from build123d import *

# Parameters (mm, degrees)
SKETCH2_R           = 11
SKETCH2_R_2         = 7
BOSS_EXTRUDE1_DEPTH = 4


with BuildPart() as part:
    # Sketch2 → Boss-Extrude1 (new body)
    with BuildSketch(Plane.XY):
        with BuildLine():
            Line((30.078103468, 30.102899094), (30.078103468, 104.858637586))
            Line((30.078103468, 104.858637586), (43.656234688, 145.478166756))
            Line((43.656234688, 145.478166756), (60.038536544, 194.486485935))
            Line((60.038536544, 194.486485935), (60.038536544, 254.427096014))
            ThreePointArc((60.038536544, 254.427096014), (45.05832001, 260.632104877), (30.078103469, 254.427096029))
            Line((30.078103469, 254.427096029), (22.62926434, 194.486485916))
            Line((22.62926434, 194.486485916), (-14.683335653, 89.230795609))
            Line((-14.683335653, 89.230795609), (-17.49123357, 0.553848547))
            ThreePointArc((-17.49123357, 0.553848547), (-3.415184823, -17.163522734), (16.370945819, -6.184022397))
            Line((16.370945819, -6.184022397), (30.078103468, 30.102899094))
        make_face()
        Circle(SKETCH2_R, mode=Mode.SUBTRACT)
        with Locations((45.058319997, 232.788133995)):
            Circle(SKETCH2_R_2, mode=Mode.SUBTRACT)
        with Locations((42.85515341, 200.574247039)):
            Circle(SKETCH2_R_2, mode=Mode.SUBTRACT)
        with Locations((32.877400798, 166.36480954)):
            Circle(SKETCH2_R_2, mode=Mode.SUBTRACT)
        with Locations((22.629264347, 133.284451418)):
            Circle(SKETCH2_R_2, mode=Mode.SUBTRACT)
        with Locations((10.792452444, 95.075946031)):
            Circle(SKETCH2_R_2, mode=Mode.SUBTRACT)
        with Locations((5.075535148, 44.712849864)):
            Circle(SKETCH2_R, mode=Mode.SUBTRACT)
    extrude(amount=BOSS_EXTRUDE1_DEPTH)


solid = part.part
Here's how the part is built. I have some questions about the finished solid (model axes, mm). Coordinates: 2 decimals unless noted, no trailing zeros. Order: outer loops, then holes, each group sorted by start corner. A loop starts at its lowest first (then second) coordinate and runs counter-clockwise, first axis right, second up.
Item 1: I need wall thicknesses on line 1 (X direction, y = 43, z = 0.2); line 2 (X direction, y = 130, z = 1.05); line 3 (X direction, y = 179.5, z = 0.2). Which ranges of each line are inside material? Lowest first, please.
Result sheet:
line 1: x = -16.15 to -5.79, 15.94 to 30.08
line 2: x = -0.23 to 16.45, 28.81 to 38.48
line 3: x = 17.32 to 55.03
Item 2: If we section it at D-D on x = -1: List the corners of the cut face in (y, z) for me, plus the area to 3 significant figures.
Result sheet:
outline: (-17.47, 0) - (-10.95, 0) - (-10.95, 4) - (-17.47, 4) - close; (10.95, 0) - (35.54, 0) - (35.54, 4) - (10.95, 4) - close; (53.88, 0) - (127.83, 0) - (127.83, 4) - (53.88, 4) - close
area: 420 mm2
Item 3: If we section it at A-A on x = 47: List the corners of the cut face in (y, z) for me, plus the area to 3 significant figures.
Result sheet:
outline: (155.48, 0) - (194.93, 0) - (194.93, 4) - (155.48, 4) - close; (206.22, 0) - (226.06, 0) - (226.06, 4) - (206.22, 4) - close; (239.51, 0) - (260.54, 0) - (260.54, 4) - (239.51, 4) - close
area: 321 mm2
Item 4: If we section it at C-C on y = 162: List the corners of the cut face in (x, z) for me.
Result sheet:
outline: (11.11, 0) - (27.4, 0) - (27.4, 4) - (11.11, 4) - close; (38.35, 0) - (49.18, 0) - (49.18, 4) - (38.35, 4) - close
Item 5: For P1, Ø1.2, axis at y = 53, z = 2, coming from the +X side, with a flat end and sliding along its axis, tell me the tip position at first contact or that it passes through.
Result sheet:
P1: stops at x = 30.08
Item 6: If we section it at B-B on z = 2.9: List the corners of the cut face in (x, y) for me.
Result sheet:
outline: (-17.49, 0.55) arc R17.5 ccw to (16.37, -6.18) - (30.08, 30.1) - (30.08, 104.86) - (60.04, 194.49) - (60.04, 254.43) arc R21.19 ccw to (30.08, 254.43) - (22.63, 194.49) - (-14.68, 89.23) - close; hole circle Ø22 at (0, 0); hole circle Ø22 at (5.08, 44.71); hole circle Ø14 at (10.79, 95.08); hole circle Ø14 at (22.63, 133.28); hole circle Ø14 at (32.88, 166.36); hole circle Ø14 at (42.86, 200.57); hole circle Ø14 at (45.06, 232.79)
Item 7: If we mould it in two halves opening along X, with no side actions, what happens to faces 1 (the face through (21.11, 126.45, 1.97)), 2 (the face through (-3.752, -17.093, 1.972)), 3 (the face through (21, 124, 0))? For each: +X half, -X half, draft (parallel to the pull), parting line (faces both ways), or undercut.
Result sheet:
face 1: undercut
face 2: parting line
face 3: draft
